Check sheet for the modelled part. Datum: model origin and axes. Units: mm. A direction names the side the tool comes from. Give positions to 0.01 mm unless a question says otherwise; leave off trailing zeros. Loops run counter-clockwise (first coordinate to the right, second up) from the corner with the lowest first, then second, coordinate; pieces in that order, holes last. Notation, with made-up numbers: (38.25, 4.5) - (50.25, 4.5) arc R10 cw to (50.25, 21.5) - close; hole circle Ø11 at (80, 23.25). An arc over 180 degrees is marked (long way). Use CSV: the item, a comma, the result in double quotes.
from build123d import *

# Parameters (mm, degrees)
SZKIC5_R                    = 51.5
DODANIE_WYCI_GNI_CIE5_DEPTH = 110
SZKIC6_R                    = 17
WYTNIJ_WYCI_GNI_CIE3_DEPTH  = 66
SZKIC8_R                    = 32
WYTNIJ_WYCI_GNI_CIE4_DEPTH  = 46
DODANIE_WYCI_GNI_CIE7_DEPTH = 22
EBRO3_START                 = -6
EBRO3_DEPTH                 = 12


# Read off the part's stored shape, not the designer's step: Żebro3
with BuildPart() as part:
    # Szkic5 → Dodanie-wyciągnięcie5 (new body)
    with BuildSketch(Plane.XY):
        Circle(SZKIC5_R)
    extrude(amount=DODANIE_WYCI_GNI_CIE5_DEPTH)

    # Szkic6 → Wytnij-wyciągnięcie3 (cut)
    with BuildSketch(Plane.XY):
        Circle(SZKIC6_R)
    extrude(amount=WYTNIJ_WYCI_GNI_CIE3_DEPTH, mode=Mode.SUBTRACT)

    # Szkic8 → Wytnij-wyciągnięcie4 (cut)
    with BuildSketch(Plane.XY.offset(110)):
        Circle(SZKIC8_R)
    extrude(amount=-WYTNIJ_WYCI_GNI_CIE4_DEPTH, mode=Mode.SUBTRACT)

    # Szkic9 → Dodanie-wyciągnięcie7 (add)
    with BuildSketch(Plane.XY.offset(110)):
        with BuildLine():
            Line((-150, 13), (-150, 38))
            Line((-150, 38), (-4.689194415, 51.286074677))
            Line((-4.689194415, 51.286074677), (4.689194415, 51.286074677))
            Line((4.689194415, 51.286074677), (150, 38))
            Line((150, 38), (150, 13))
            Line((150, 13), (105, 13))
            ThreePointArc((105, 13), (92, 0), (105, -13))
            Line((105, -13), (150, -13))
            Line((150, -13), (150, -38))
            Line((150, -38), (4.689194415, -51.286074677))
            Line((4.689194415, -51.286074677), (-4.689194415, -51.286074677))
            Line((-4.689194415, -51.286074677), (-150, -38))
            Line((-150, -38), (-150, -13))
            Line((-150, -13), (-105, -13))
            ThreePointArc((-105, -13), (-92, 0), (-105, 13))
            Line((-105, 13), (-150, 13))
        make_face()
    extrude(amount=-DODANIE_WYCI_GNI_CIE7_DEPTH)

    # Żebro3 outline → Żebro3 (add)
    with BuildSketch(Plane(origin=(0, 0, 0), x_dir=(1, 0, 0), z_dir=(0, 1, 0)).offset(EBRO3_START)):
        Polygon((66.136905435, -88), (51.5, 0), (51, 0), (51, -89), (66.303233906, -89), align=None)
    ebro3 = extrude(amount=EBRO3_DEPTH)

    # Lustro2: Żebro3 across plane
    add(ebro3.mirror(Plane(origin=(0, 0, 0), x_dir=(0, 0, 1), z_dir=(1, 0, 0))))


solid = part.part
1. Set-up check for faces 4 (the face through (57, 6, 53)), 5 (the face through (1.05, 51.49, 42.01)), 6 (the face through (-127, 13, 99)), 7 (the face through (57, -6, 53)), 8 (the face through (0, 0, 88)): record each of +Z, -Z, +X, -X, +Y, -Y from which the full face is reachable in a straight line by a thin tool's end or side.
Completed:
face 4,"-Z, +X, +Y"
face 5,"-Z, +Y"
face 6,"+Z, -Z, -X"
face 7,"-Z, +X, -Y"
face 8,"none"
2. Sectioned sample at C-C, the plane x = -128.5. Record the boundary of the cut face in (y, z).
Completed:
outline,"(-39.97, 88) - (-13, 88) - (-13, 110) - (-39.97, 110) - close; (13, 88) - (39.97, 88) - (39.97, 110) - (13, 110) - close"
3. Sectioned sample at A-A, the plane x = 0. Record the boundary of the cut face in (y, z), and give its area (3 significant figures).
Completed:
outline,"(-51.5, 0) - (-17, 0) - (-17, 64) - (-32, 64) - (-32, 88) - (32, 88) - (32, 64) - (17, 64) - (17, 0) - (51.5, 0) - (51.5, 110) - (-51.5, 110) - close"
area,"7,620 mm²"
4. Sectioned sample at D-D, the plane y = 0. Record the boundary of the cut face in (x, z), and give its area (3 significant figures).
Completed:
outline,"(-92, 88) - (-66.14, 88) - (-51.5, 0) - (-17, 0) - (-17, 64) - (-32, 64) - (-32, 88) - (32, 88) - (32, 64) - (17, 64) - (17, 0) - (51.5, 0) - (66.14, 88) - (92, 88) - (92, 110) - (-92, 110) - close"
area,"10,700 mm²"
5. Release check for a two-part mould opening along X. For faces 1 (the face through (92, 0, 99)), 2 (the face through (-6.94, -31.24, 76.17)), 3 (the face through (-92, 0, 99)) record: released by +X, released by -X, zero draft, split by the parting line, or undercut.
Completed:
face 1,"released by +X"
face 2,"undercut"
face 3,"released by -X"
6. Sectioned sample at B-B, the plane y = 27.5. Record the boundary of the cut face in (x, z), and give its area (3 significant figures).
Completed:
outline,"(-150, 88) - (-43.54, 88) - (-43.54, 0) - (43.54, 0) - (43.54, 88) - (150, 88) - (150, 110) - (-150, 110) - close; hole (-16.36, 64) - (16.36, 64) - (16.36, 88) - (-16.36, 88) - close"
area,"13,500 mm²"
7. Go/stop test with flat-tipped pins: pin 1 Ø12 at (y, z) = (-2.5, 67) entering from +X; pin 2 Ø17.5 at (x, z) = (121, 104) entering from +Y; pin 3 Ø11 at (x, z) = (-124, 99.5) entering from +Y. Record where each tip stops, or that it passes through.
Completed:
pin 1,"stops at x = 63.64"
pin 2,"stops at y = 41.45"
pin 3,"stops at y = 40.88"
8. Scan lines: line 1 along Y through (x, z) = (0, 73.5); line 2 along Y through (x, z) = (0, 29); line 3 along Z through (x, y) = (14, -19.5). Record each from-to range of solid material in increasing order.
Completed:
line 1,"y = -51.5 to -32, 32 to 51.5"
line 2,"y = -51.5 to -17, 17 to 51.5"
line 3,"z = 0 to 64, 88 to 110"
